The listing builds one solid part. Answer for the finished solid, in the listing's coordinates (mm). A direction names the side the tool comes from. Give positions to 0.01 mm unless a question says otherwise; leave off trailing zeros. Write each loop counter-clockwise with the first axis right and the second up, starting at its lowest first coordinate (ties: lowest second). Pieces come first, ordered by that corner, then holes. Notation, with made-up numbers: (7.5, -26.75) -> (57.5, -26.75) arc R27 ccw to (57.5, -3.75) -> close; hole circle Ø4 at (34, 7). An arc over 180 degrees is marked (long way). Use CSV: the item, a comma, the result in double quotes. Start each with the question number.
Autodesk Inventor part; units mm, degrees
ref_plane "YZ Plane" through (0, 0, 0) normal (1, 0, 0) x (0, 1, 0)
ref_plane "XZ Plane" through (0, 0, 0) normal (0, 1, 0) x (-1, 0, 0)
ref_plane "XY Plane" through (0, 0, 0) normal (0, 0, 1) x (1, 0, 0)
sketch "Sketch1" plane through (0, 0, 0) normal (0, 0, 1) x (1, 0, 0)
  line L0 (0, 0) -> (68, 0)
  line L1 (68, 0) -> (68, 48)
  line L2 (68, 48) -> (0, 48)
  line L3 (0, 48) -> (0, 0)
  dimension "d0" = 68
  dimension "d1" = 48
extrude "Extrusion1" add sketch "Sketch1" along normal blind 2
sketch "Sketch2" plane through (0, 0, 2) normal (0, 0, 1) x (1, 0, 0)
  circle A0 centre (6.2, 37) radius 2.4
  circle A1 centre (61.8, 37) radius 2.4
  line L0 (0, 0) -> (68, 0)
  line L1 (34, 0) -> (34, 48) construction
  line L2 (68, 48) -> (0, 48)
  dimension "d4" = 4.8
  dimension "d5" = 4.8
  dimension "d6" = 55.6
  dimension "d7" = 27.8
  dimension "d8" = 37
extrude "Extrusion2" cut sketch "Sketch2" against normal blind 2
sketch "Sketch3" plane through (0, 0, 0) normal (0, 0, -1) x (-1, 0, 0)
  line L0 (-68, 48) -> (0, 48)
  line L1 (0, 48) -> (0, 46)
  line L2 (0, 46) -> (-68, 46)
  line L3 (-68, 46) -> (-68, 48)
  line L4 (0, 0) -> (0, 2)
  line L5 (-68, 2) -> (-68, 0)
  dimension "d11" = 2
extrude "Extrusion3" add sketch "Sketch3" along normal blind 18
properties part number "MainsCover"
Q1. Section A-A on x = 61.8 is taken. Give the vertices of the cut face in (y, z).
Q2. Section C-C on x = 42 is taken. Give the vertices of the cut face in (y, z).
Q3. For faces 5 (the face through (34, 24, 2)), 6 (the face through (34, 23, 0)), determine the directions among +Z, -Z, +X, -X, +Y, -Y from which every point of the face is accessible in a straight line to the end or side of a thin tool.
Q4. Section D-D on y = 27 is taken. Give the vertices of the cut face in (x, z).
Q5. Section B-B on y = 37 is taken. Give the vertices of the cut face in (x, z), then the cut area to 3 significant figures.
Q6. The mould has two halves that part along Y. Classify faces 1 (the face through (34, 46, -9)), 2 (the face through (5.68, 34.657, 1.014)), 3 (the face through (68, 27.4, 0.2)), 4 (the face through (61.28, 34.657, 1.014)): +Y half, -Y half, draft (parallel to the pull), parting line (faces both ways), or undercut.
Q7. Flat-ended cylindrical pins translate along their axes: pin 1 Ø2 at (x, z) = (53.5, -3.5) entering from -Y; pin 2 Ø12 at (x, y) = (13.5, 39) entering from -Z. Find the tip coordinate at first contact, or state that the pin passes through.
Q8. Straight lines are drawn through the part: L1, parallel to Y at x = 61.8, z = 1.65; L2, parallel to Z at x = 44.5, y = 41; L3, parallel to Y at x = 6, z = -10.5. For each, find the intervals that lie inside material, in ascending order.
Output:
1,outline,"(0, 0) -> (34.6, 0) -> (34.6, 2) -> (0, 2) -> close; (39.4, 0) -> (46, 0) -> (46, -18) -> (48, -18) -> (48, 2) -> (39.4, 2) -> close"
2,outline,"(0, 0) -> (46, 0) -> (46, -18) -> (48, -18) -> (48, 2) -> (0, 2) -> close"
3,face 5,"+Z, +X, -X, +Y, -Y"
3,face 6,"-Z, +X, -X, -Y"
4,outline,"(0, 0) -> (68, 0) -> (68, 2) -> (0, 2) -> close"
5,outline,"(0, 0) -> (3.8, 0) -> (3.8, 2) -> (0, 2) -> close; (8.6, 0) -> (59.4, 0) -> (59.4, 2) -> (8.6, 2) -> close; (64.2, 0) -> (68, 0) -> (68, 2) -> (64.2, 2) -> close"
5,area,"117 mm²"
6,face 1,"-Y half"
6,face 2,"undercut"
6,face 3,"draft"
6,face 4,"undercut"
7,pin 1,"y = 46"
7,pin 2,"z = 0"
8,L1,"0 to 34.6, 39.4 to 48"
8,L2,"0 to 2"
8,L3,"46 to 48"
